from build123d import *

# Parameters (mm, degrees)
PAD_DEPTH    = 25
SKETCH001_R  = 3.075
PAD001_DEPTH = 1.7
SKETCH011_R  = 5
PAD009_DEPTH = 4


with BuildPart() as part:
    # Sketch → Pad (new body)
    with BuildSketch(Plane.XZ):
        with BuildLine():
            Line((-6.63325, 7.55), (6.63325, 7.55))
            ThreePointArc((6.63325, -7.55), (10.05, 0), (6.63325, 7.55))
            Line((6.63325, -7.55), (-6.63325, -7.55))
            ThreePointArc((-6.63325, 7.55), (-10.05, 0), (-6.63325, -7.55))
        make_face()
    extrude(amount=PAD_DEPTH)

    # Sketch001 → Pad001 (new body)
    with BuildSketch(Plane.XZ.offset(25)):
        Circle(SKETCH001_R)
    extrude(amount=PAD001_DEPTH)

    # Sketch011 → Pad009 (new body)
    with BuildSketch(Plane(origin=(0, 0, 0), x_dir=(1, 0, 0), z_dir=(0, 1, 0))):
        Circle(SKETCH011_R)
    extrude(amount=PAD009_DEPTH)


solid = part.part
The model under review builds one solid part; all positions refer to its coordinate system, in mm. A direction names the side the tool comes from. Round coordinates to 2 decimals unless told otherwise and drop trailing zeros. Write each loop counter-clockwise with the first axis right and the second up, starting at its lowest first coordinate (ties: lowest second). Pieces come first, ordered by that corner, then holes. Notation, with made-up numbers: (29.25, 53) - (75.25, 53) arc R31 ccw to (75.25, 92) - close; hole circle Ø10 at (49.5, -11.5). An arc over 180 degrees is marked (long way). One line per item, written item: value. Start each with the question number.
1. To check wall thickness, follow L1, parallel to Y at x = 5.5, z = -2.75; L2, parallel to Y at x = 2.75, z = 2.25; L3, parallel to X at y = 2, z = 4.25. State the ranges of each line that lie inside material, in increasing order. Write a range as from..to.
2. Consider section C-C on y = -16. Write out the cut boundary in (x, z), and give its area (3 significant figures).
3. Consider section D-D on x = 0. Write out the cut boundary in (y, z) (3 decimals).
4. Consider section A-A on z = 0. Write out the cut boundary in (x, y) (3 decimals), and give its area (3 significant figures).
5. Machinability: for faces 1 (the face through (0, 4, 0)), 2 (the face through (-1.08, 1.97, 4.88)), 3 (the face through (-0.67, -25.84, -3)), which of the approach directions +Z, -Z, +X, -X, +Y, -Y give a long, thin tool a straight path to every point of the face, cutting with its end or side? Answer none if there is none.
6. Clearance check with a flat-ended pin moving along its axis: P1, Ø6, axis at y = -15, z = 5, coming from the -X side. State where the tip first meets the part, or that it passes through.
7. Consider section B-B on x = 4. Write out the cut boundary in (y, z).
Checks:
1. L1: y = -25..0
1. L2: y = -25..4
1. L3: x = -2.63..2.63
2. outline: (-6.63, -7.55) - (6.63, -7.55) arc R10.05 ccw to (6.63, 7.55) - (-6.63, 7.55) arc R10.05 ccw to start
2. area: 272 mm^2
3. outline: (-26.7, -3.075) - (-25, -3.075) - (-25, -7.55) - (0, -7.55) - (0, -5) - (4, -5) - (4, 5) - (0, 5) - (0, 7.55) - (-25, 7.55) - (-25, 3.075) - (-26.7, 3.075) - close
4. outline: (-10.05, -25) - (-3.075, -25) - (-3.075, -26.7) - (3.075, -26.7) - (3.075, -25) - (10.05, -25) - (10.05, 0) - (5, 0) - (5, 4) - (-5, 4) - (-5, 0) - (-10.05, 0) - close
4. area: 553 mm^2
5. face 1: +Z, -Z, +X, -X, +Y
5. face 2: +Y
5. face 3: -Y
6. P1: stops at x = -9.85
7. outline: (-25, -7.55) - (0, -7.55) - (0, -3) - (4, -3) - (4, 3) - (0, 3) - (0, 7.55) - (-25, 7.55) - close
